CAD build for the part. Positions are in the model's coordinates, mm. A direction names the side the tool comes from. Coordinates: 2 decimals unless noted, no trailing zeros. Order: outer loops, then holes, each group sorted by start corner. A loop starts at its lowest first (then second) coordinate and runs counter-clockwise, first axis right, second up.
from build123d import *

# Parameters (mm, degrees)
F0_W         = 100
F0_H         = 50
F1_DEPTH     = 25
F3_W         = 44
F3_H         = 20
F4_DEPTH     = 100.001
F2_W         = 94
F2_H         = 20
F5_DEPTH     = 50.001
F6_W         = 94
F6_H         = 44
F6_H_2       = 0.75
F7_DEPTH     = 2.5
F8_DEPTH     = 3
F2_H_2       = 2.5
F9_DEPTH     = 0.75
F10_W        = 44
F10_H        = 2.5
F11_DEPTH    = 0.75
F13_DEPTH    = 0.75
F14_W        = 44
F14_H        = 2.5
F15_DEPTH    = 0.75
F16_W        = 44
F16_H        = 2.5
F17_DEPTH    = 0.75
F18_W        = 94
F18_H        = 2.5
F19_DEPTH    = 0.75
F20_W        = 94
F20_H        = 2.5
F21_DEPTH    = 0.75
F22_T1_DEPTH = 75
F22_T3_DEPTH = 125


# Not quite as in the source:
# - a fillet or chamfer that OpenCascade refuses, or shapes differently, is made with other operations: its cross-section is extruded or revolved along the edge and cut away or added


with BuildPart() as f1:
    # F0 (on Top) → F1 (new body)
    with BuildSketch(Plane.XY):
        with Locations((50, 25)):
            Rectangle(F0_W, F0_H)
    extrude(amount=F1_DEPTH)

    # F3 (on face) → F4 (cut, through all)
    with BuildSketch(Plane.YZ.offset(100)):
        with Locations((25, 10)):
            Rectangle(F3_W, F3_H)
    extrude(amount=-F4_DEPTH, mode=Mode.SUBTRACT)

    # F2 (on face) → F5 (cut, through all)
    with BuildSketch(Plane.XZ):
        with Locations((50, 10)):
            Rectangle(F2_W, F2_H)
    extrude(amount=-F5_DEPTH, mode=Mode.SUBTRACT)

    # F6 (on face) → F7 (cut)
    with BuildSketch(Plane(origin=(0, 0, 20), x_dir=(1, 0, 0), z_dir=(0, 0, -1))):
        with Locations((50, -25)):
            Rectangle(F6_W, F6_H)
        with Locations((50, -2.625)):
            Rectangle(F6_W, F6_H_2)
    extrude(amount=-F7_DEPTH, mode=Mode.SUBTRACT)

    # F6 (on face) → F8 (cut)
    with BuildSketch(Plane(origin=(0, 0, 20), x_dir=(1, 0, 0), z_dir=(0, 0, -1))):
        with Locations((50, -25)):
            Rectangle(F6_W, F6_H)
    extrude(amount=-F8_DEPTH, mode=Mode.SUBTRACT)

    # F2 (on face) → F9 (cut)
    with BuildSketch(Plane.XZ):
        with Locations((50, 21.25)):
            Rectangle(F2_W, F2_H_2)
    extrude(amount=-F9_DEPTH, mode=Mode.SUBTRACT)

    # F10 (on face) → F11 (cut)
    with BuildSketch(Plane(origin=(0, 0, 0), x_dir=(0, -1, 0), z_dir=(-1, 0, 0))):
        with Locations((-25, 21.25)):
            Rectangle(F10_W, F10_H)
    extrude(amount=-F11_DEPTH, mode=Mode.SUBTRACT)

    # F12 (on face) → F13 (cut)
    with BuildSketch(Plane.YZ.offset(3)):
        Polygon((3, 22.5), (3, 20), (47, 20), (47, 21.5), (47, 22.5), align=None)
    extrude(amount=-F13_DEPTH, mode=Mode.SUBTRACT)

    # F14 (on face) → F15 (cut)
    with BuildSketch(Plane.YZ.offset(100)):
        with Locations((25, 21.25)):
            Rectangle(F14_W, F14_H)
    extrude(amount=-F15_DEPTH, mode=Mode.SUBTRACT)

    # F16 (on face) → F17 (cut)
    with BuildSketch(Plane(origin=(97, 0, 0), x_dir=(0, -1, 0), z_dir=(-1, 0, 0))):
        with Locations((-25, 21.25)):
            Rectangle(F16_W, F16_H)
    extrude(amount=-F17_DEPTH, mode=Mode.SUBTRACT)

    # F18 (on face) → F19 (cut)
    with BuildSketch(Plane(origin=(0, 50, 0), x_dir=(-1, 0, 0), z_dir=(0, 1, 0))):
        with Locations((-50, 21.25)):
            Rectangle(F18_W, F18_H)
    extrude(amount=-F19_DEPTH, mode=Mode.SUBTRACT)

    # F20 (on face) → F21 (cut)
    with BuildSketch(Plane.XZ.offset(-47)):
        with Locations((50, 21.25)):
            Rectangle(F20_W, F20_H)
    extrude(amount=-F21_DEPTH, mode=Mode.SUBTRACT)

    # F22: fillet of radius 5 on 4 edges, made by hand

    # F22_s2 → F22_t1 (cut)
    with BuildSketch(Plane.XZ.offset(-62.5)):
        with BuildLine():
            ThreePointArc((0, 20), (1.4644660941, 23.5355339059), (5, 25))
            Line((5, 25), (0, 25))
            Line((0, 25), (0, 20))
        make_face()
        with BuildLine():
            ThreePointArc((100, 20), (98.5355339059, 23.5355339059), (95, 25))
            Line((95, 25), (100, 25))
            Line((100, 25), (100, 20))
        make_face()
    extrude(amount=F22_T1_DEPTH, mode=Mode.SUBTRACT)

    # F22_s4 → F22_t3 (cut)
    with BuildSketch(Plane.YZ.offset(-12.5)):
        with BuildLine():
            ThreePointArc((0, 20), (1.4644660941, 23.5355339059), (5, 25))
            Line((5, 25), (0, 25))
            Line((0, 25), (0, 20))
        make_face()
        with BuildLine():
            ThreePointArc((45, 25), (48.5355339059, 23.5355339059), (50, 20))
            Line((50, 20), (50, 25))
            Line((50, 25), (45, 25))
        make_face()
    extrude(amount=F22_T3_DEPTH, mode=Mode.SUBTRACT)


solid = f1.part
1) Pin check, flat tips, straight feed: P1, Ø2, axis at x = 62, z = 18.5, coming from the -Y side; P2, Ø2, axis at x = 42, y = 43.5, coming from the -Z side; P3, Ø0.6, axis at x = 66.5, y = 47.5, coming from the -Z side; P4, Ø4, axis at y = 11, z = 22, coming from the +X side. Stop position of each tip, or through.
2) Drill centre lines: probe 1 along X at (y, z) = (2, 13.25); probe 2 along Y at (x, z) = (16, 22); probe 3 along Z at (x, y) = (57, 41.5). Where is each one in solid material? Low to high.
3) Slice it at C-C (y = 6). List the corners of the cut face in (x, z).
4) Slice it at B-B (x = 50.5). List the corners of the cut face in (y, z).
5) Which spindle directions (+Z, -Z, +X, -X, +Y, -Y) get a long thin tool onto all of the face, cutting with end or side? Do faces 5 (the flat face through (49, 2.25, 21)), 6 (the flat face through (99.25, 25, 21)), 7 (the flat face through (0, 48, 10)), 8 (the flat face through (49, 0.75, 21)), 9 (the flat face through (49, 25, 25)). Say none if no direction does.
6) Slice it at A-A (z = 18.5). List the corners of the cut face in (x, y), plus the area to 3 significant figures.
7) Two-plate mould, pull along Y, no slides. Class faces 1 (the flat face through (98, 2, 0)), 2 (the flat face through (97.75, 25, 21)), 3 (the flat face through (98, 50, 10)), 4 (the flat face through (0.75, 25, 21)): released by +Y, released by -Y, zero draft, split by the parting line, or undercut.
Worked out:
1. P1: passes through
1. P2: stops at z = 23
1. P3: stops at z = 20
1. P4: stops at x = 99.33
2. probe 1: x = 0 to 3, 97 to 100
2. probe 2: y = 0.75 to 2.25, 47.75 to 49.25
2. probe 3: z = 23 to 25
3. outline: (0.67, 22.5) - (0.75, 22.5) - (0.75, 20) - (2.25, 20) - (2.25, 22.5) - (3, 22.5) - (3, 23) - (97, 23) - (97, 22.5) - (97.75, 22.5) - (97.75, 20) - (99.25, 20) - (99.25, 22.5) - (99.33, 22.5) arc R5 ccw to (95, 25) - (5, 25) arc R5 ccw to start
4. outline: (0.67, 22.5) - (0.75, 22.5) - (0.75, 20) - (2.25, 20) - (2.25, 22.5) - (3, 22.5) - (3, 23) - (47, 23) - (47, 22.5) - (47.75, 22.5) - (47.75, 20) - (49.25, 20) - (49.25, 22.5) - (49.33, 22.5) arc R5 ccw to (45, 25) - (5, 25) arc R5 ccw to start
5. face 5: -Z
5. face 6: -Z, +X
5. face 7: +Z, -Z, -X, +Y, -Y
5. face 8: -Z, -Y
5. face 9: +Z, +X, -X, +Y, -Y
6. outline: (0, 0) - (3, 0) - (3, 3) - (0, 3) - close; (0, 47) - (3, 47) - (3, 50) - (0, 50) - close; (97, 0) - (100, 0) - (100, 3) - (97, 3) - close; (97, 47) - (100, 47) - (100, 50) - (97, 50) - close
6. area: 36.0 mm2
7. face 1: zero draft
7. face 2: undercut
7. face 3: released by +Y
7. face 4: undercut
